from build123d import *

# Parameters (mm, degrees)
BOSS_EXTRUDE1_DEPTH = 15
SHELL3_DEPTH        = 13.5
SKETCH5_R           = 18
CUT_EXTRUDE4_DEPTH  = 11
BOSS_EXTRUDE2_START = -8
BOSS_EXTRUDE2_DEPTH = 7
CUT_EXTRUDE5_REACH  = 54.505


# Read off the part's stored shape, not the designer's step: Shell3
with BuildPart() as part:
    # Sketch1 → Boss-Extrude1 (new body)
    with BuildSketch(Plane.XY):
        with BuildLine():
            Line((-7.603827524, -22.477243695), (7.603827524, -22.477243695))
            Line((7.603827524, -22.477243695), (14.409989224, -15.275870207))
            ThreePointArc((14.409989224, -15.275870207), (0, 21), (-14.409989224, -15.275870207))
            Line((-14.409989224, -15.275870207), (-7.603827524, -22.477243695))
        make_face()
    extrude(amount=BOSS_EXTRUDE1_DEPTH)

    # Shell3 outline → Shell3 (cut)
    with BuildSketch(Plane.XY):
        with BuildLine():
            Line((6.863063192, -21.077243695), (13.349946464, -14.213688101))
            ThreePointArc((13.349946464, -14.213688101), (0, 19.5), (-13.349946464, -14.213688101))
            Line((-13.349946464, -14.213688101), (-6.863063192, -21.077243695))
            Line((-6.863063192, -21.077243695), (6.863063192, -21.077243695))
        make_face()
    extrude(amount=SHELL3_DEPTH, mode=Mode.SUBTRACT)

    # Sketch5 → Cut-Extrude4 (cut)
    with BuildSketch(Plane.XY.offset(15)):
        Circle(SKETCH5_R)
    extrude(amount=-CUT_EXTRUDE4_DEPTH, mode=Mode.SUBTRACT)

    # Sketch6 → Boss-Extrude2 (add)
    with BuildSketch(Plane.XY.offset(15).offset(BOSS_EXTRUDE2_START)):
        Polygon((17.530464007, 10.991223826), (24.980464007, 10.991223826), (24.980464007, 5.991223826), (19.980464007, 5.991223826), align=None)
        Polygon((17.673562003, -11.090259794), (20.075985217, -6.005149393), (25.123075828, -6.005149393), (25.123075828, -11.005149393), align=None)
        Polygon((-17.877308509, 10.991223826), (-20.094018297, 5.991223826), (-25.327308509, 5.991223826), (-25.327308509, 10.991223826), align=None)
        Polygon((-25.294081514, -11.005149393), (-25.294081514, -6.005149393), (-20.094018297, -6.005149393), (-17.844081514, -11.005149393), align=None)
    extrude(amount=-BOSS_EXTRUDE2_DEPTH)

    # Sketch21 → Cut-Extrude5 (cut, up to next)
    with BuildSketch(Plane.XZ.offset(22.477243695), mode=Mode.PRIVATE) as cut_extrude5_sk1:
        with BuildLine():
            Line((-3.249172698, 8.75), (3.250827302, 8.75))
            ThreePointArc((3.250827302, 8.75), (4.750827302, 7.25), (3.250827302, 5.75))
            Line((3.250827302, 5.75), (-3.249172698, 5.75))
            ThreePointArc((-3.249172698, 5.75), (-4.749172698, 7.25), (-3.249172698, 8.75))
        make_face()
    cut_extrude5_tool1 = extrude(cut_extrude5_sk1.sketch, amount=-CUT_EXTRUDE5_REACH, mode=Mode.PRIVATE) & part.part
    add(cut_extrude5_tool1.solids().sort_by_distance((0.000827, -22.477244, 7.25))[0], mode=Mode.SUBTRACT)


solid = part.part
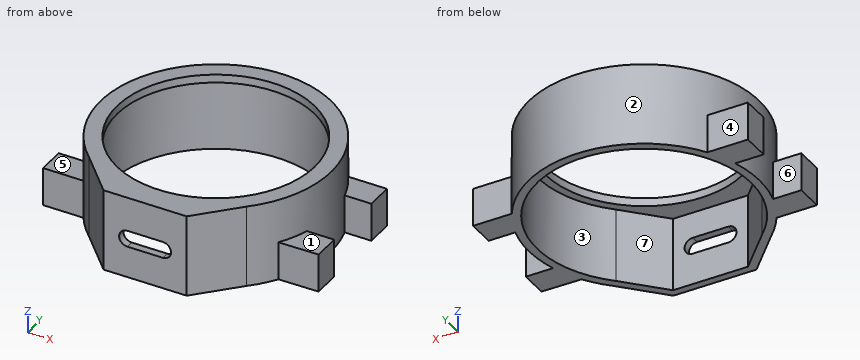
Design review of the part built by this model. Coordinates are the model's own, in mm. Face numbers are marked on the shaded views. A direction names the side the tool comes from. Give positions to 0.01 mm unless a question says otherwise; leave off trailing zeros. Loops run counter-clockwise (first coordinate to the right, second up) from the corner with the lowest first, then second, coordinate; pieces in that order, holes last. Notation, with made-up numbers: M 71.25,61.5 L 121.25,61.5 A21 cw 121.25,70.5 Z; hole C -32.5,20.5 d4. An arc over 180 degrees is marked long. One line per question, with ' | ' between items. Start each with the question number.
1. To check wall thickness, follow L1, parallel to X at y = 0, z = 10; L2, parallel to Y at x = 0, z = 13.9; L3, parallel to Z at x = 2.5, y = 18. State the ranges of each line that lie inside material, in increasing order.
2. Insertion check: P1, Ø4, axis at x = 12.5, z = 4, coming from the +Y side; P2, Ø8, axis at y = 6.5, z = 5, coming from the +X side; P3, Ø5, axis at y = 14, z = 8.5, coming from the -X side. Each pin has a flat end and moves straight along its axis. Give the tip position at first contact, or say it passes through.
3. Add section C-C (x = 0). Write out the cut boundary in (y, z).
4. Add section B-B (z = 11.5). Write out the cut boundary in (x, y).
5. The part is to be moulded in two halves that separate along X. For the marked faces 1, 2 and 3, say which applies: released by +X, released by -X, zero draft, split by the parting line, or undercut.
6. Add section A-A (y = 0). Write out the cut boundary in (x, z), plus the area to 3 significant figures.
7. For the marked faces 4, 5, 6 and 7, list the 3-axis set-ups (+Z, -Z, +X, -X, +Y, -Y) from which the entire face can be reached by the end or side of a thin tool; tool diameter is ignored.
8. Add section D-D (x = 15). Write out the cut boundary in (y, z), plus the area to 3 significant figures.
Worked out:
1) L1: x = -21 to -19.5, 19.5 to 21 | L2: y = -22.48 to -18, 18 to 21 | L3: z = 13.5 to 15
2) P1: stops at y = 18.19 | P2: stops at x = 24.98 | P3: stops at x = -17.57
3) outline: M -22.48,0 L -21.08,0 L -21.08,5.75 L -22.48,5.75 Z; M -22.48,8.75 L -21.08,8.75 L -21.08,13.5 L -18,13.5 L -18,15 L -22.48,15 Z; M 18,13.5 L 19.5,13.5 L 19.5,0 L 21,0 L 21,15 L 18,15 Z
4) outline: M -14.41,-15.28 L -7.6,-22.48 L 7.6,-22.48 L 14.41,-15.28 A21 ccw long Z; hole M -13.35,-14.21 L -6.86,-21.08 L 6.86,-21.08 L 13.35,-14.21 A19.5 ccw long Z
5) face 1: zero draft | face 2: split by the parting line | face 3: undercut
6) outline: M -21,0 L -19.5,0 L -19.5,13.5 L -18,13.5 L -18,15 L -21,15 Z; M 18,13.5 L 19.5,13.5 L 19.5,0 L 21,0 L 21,15 L 18,15 Z | area: 49.5 mm²
7) face 4: +Z, -Z, -X, +Y | face 5: +Z, -X, -Y | face 6: +Z, -Z, -X | face 7: -Z
8) outline: M -14.7,0 L -12.46,0 L -12.46,13.5 L -9.95,13.5 L -9.95,15 L -14.7,15 Z; M 9.95,13.5 L 12.46,13.5 L 12.46,0 L 14.7,0 L 14.7,15 L 9.95,15 Z | area: 74.6 mm²
